Part model, mm, in its own coordinate system. A direction names the side the tool comes from. Round coordinates to 2 decimals unless told otherwise and drop trailing zeros. Loops run counter-clockwise (first coordinate to the right, second up) from the corner with the lowest first, then second, coordinate; pieces in that order, holes last. Notation, with made-up numbers: (79.25, 3) - (90.25, 3) arc R30 ccw to (90.25, 42) - close; hole circle Ø3 at (43, -35.75). An arc over 180 degrees is marked (long way). Write each question's results on one line, items separated by ' | '. Start each with the question number.
(1) Cut at A-A, the plane y = 8.25. List the corners of the cut face in (x, z), then the cut area to 3 significant figures.
(2) Cut at C-C, the plane z = -9. List the corners of the cut face in (x, y), then the cut area to 3 significant figures.
(3) Tool access for faces 4 (the face through (0, 6, -1)), 5 (the face through (-29, 7, 1)): list every direction of +Z, -Z, +X, -X, +Y, -Y with a clear straight run to the whole face (end or side of a thin tool).
(4) Cut at D-D, the plane y = 16.25. List the corners of the cut face in (x, z), then the cut area to 3 significant figures.
(5) Mould opens along Z. For faces 1 (the face through (0, 12, -44)), 2 (the face through (28.14, 8.63, -45.1)), 3 (the face through (0, 0, -1)) say: released by +Z, released by -Z, zero draft, split by the parting line, or undercut.
(6) Cut at B-B, the plane x = -24. List the corners of the cut face in (y, z).
(7) Drill centre lines: L1, parallel to Z at x = -24, y = 15.25; L2, parallel to X at y = 14.75, z = -16; L3, parallel to Y at x = 25, z = 38. Where is each one in solid material? Low to high.
from build123d import *

# Parameters (mm, degrees)
SKETCH1_W           = 58
SKETCH1_H           = 92
BOSS_EXTRUDE1_DEPTH = 17.5
SKETCH2_W           = 54
SKETCH2_H           = 88
CUT_EXTRUDE1_DEPTH  = 11.5
FILLET3_R           = 3


with BuildPart() as part:
    # Sketch1 → Boss-Extrude1 (new body)
    with BuildSketch(Plane(origin=(0, 0, 0), x_dir=(1, 0, 0), z_dir=(0, 1, 0))):
        Rectangle(SKETCH1_W, SKETCH1_H)
    extrude(amount=BOSS_EXTRUDE1_DEPTH)

    # Sketch2 → Cut-Extrude1 (cut)
    with BuildSketch(Plane(origin=(0, 17.5, 0), x_dir=(1, 0, 0), z_dir=(0, 1, 0))):
        Rectangle(SKETCH2_W, SKETCH2_H)
    extrude(amount=-CUT_EXTRUDE1_DEPTH, mode=Mode.SUBTRACT)

    # Fillet3
    # the kernel refuses this fillet: 3 mm, written as the material it takes off along each edge
    with BuildSketch(Plane(origin=(29, -7.5, -46), x_dir=(0, 0, 1), z_dir=(0, 1, 0)), Plane(origin=(29, -7.5, 46), x_dir=(-1, 0, 0), z_dir=(0, 1, 0))) as fillet3_piece_1:
        with BuildLine():
            CenterArc((FILLET3_R, -FILLET3_R), FILLET3_R, 90, 90)
            Line((0, -FILLET3_R), (0, 0))
            Line((0, 0), (FILLET3_R, 0))
        make_face()
    extrude(amount=32.5, mode=Mode.SUBTRACT)
    with BuildSketch(Plane(origin=(29, 17.5, 53.5), x_dir=(0, -1, 0), z_dir=(0, 0, -1)), Plane(origin=(-29, 17.5, -53.5), x_dir=(0, -1, 0), z_dir=(0, 0, 1))) as fillet3_piece_2:
        with BuildLine():
            CenterArc((FILLET3_R, FILLET3_R), FILLET3_R, 180, 90)
            Line((0, FILLET3_R), (0, 0))
            Line((0, 0), (FILLET3_R, 0))
        make_face()
    extrude(amount=107, mode=Mode.SUBTRACT)
    with BuildSketch(Plane(origin=(-29, -7.5, -46), x_dir=(0, 0, 1), z_dir=(0, 1, 0)), Plane(origin=(-29, -7.5, 46), x_dir=(1, 0, 0), z_dir=(0, 1, 0))) as fillet3_piece_3:
        with BuildLine():
            CenterArc((FILLET3_R, FILLET3_R), FILLET3_R, 180, 90)
            Line((0, FILLET3_R), (0, 0))
            Line((0, 0), (FILLET3_R, 0))
        make_face()
    extrude(amount=32.5, mode=Mode.SUBTRACT)


solid = part.part
A:
1) outline: (-29, -43) arc R3 ccw to (-26, -46) - (26, -46) arc R3 ccw to (29, -43) - (29, 43) arc R3 ccw to (26, 46) - (-26, 46) arc R3 ccw to (-29, 43) - close; hole (-27, -44) - (27, -44) - (27, 44) - (-27, 44) - close | area: 576 mm2
2) outline: (-29, 0) - (29, 0) - (29, 14.5) arc R3 ccw to (27, 17.33) - (27, 6) - (-27, 6) - (-27, 17.33) arc R3 ccw to (-29, 14.5) - close | area: 390 mm2
3) face 4: +Y | face 5: +Z, -Z, -X, +Y, -Y
4) outline: (-28.44, -44.75) arc R3 ccw to (-26, -46) - (26, -46) arc R3 ccw to (28.44, -44.75) - (28.44, 44.75) arc R3 ccw to (26, 46) - (-26, 46) arc R3 ccw to (-28.44, 44.75) - close; hole (-27, -44) - (27, -44) - (27, 44) - (-27, 44) - close | area: 477 mm2
5) face 1: undercut | face 2: released by -Z | face 3: zero draft
6) outline: (0, -46) - (17.5, -46) - (17.5, -44) - (6, -44) - (6, 44) - (17.5, 44) - (17.5, 46) - (0, 46) - close
7) L1: -46 to -44, 44 to 46 | L2: -28.99 to -27, 27 to 28.99 | L3: 0 to 6
